```python
from build123d import *

# Parameters (mm, degrees)
F1_DEPTH  = 25.4
F2_R      = 6.2243902107
F2_R_2    = 6.3495156859
F3_DEPTH  = 12.701
F6_DEPTH  = 12.701
F8_DEPTH  = 12.701
F10_DEPTH = 12.701
F11_DEPTH = 12.701
F12_DEPTH = 12.701


# Not quite as in the source:
# - a feature names something its author has since deleted; it is built from what else it names


with BuildPart() as f1:
    # F0 (on Front) → F1 (new body)
    with BuildSketch(Plane.XZ):
        Polygon((-18.3063060958, 44.45), (-31.0063060958, 44.45), (-31.0063060958, 0), (26.1436939042, 0), (26.1436939042, 12.7), (-18.3063060958, 12.7), align=None)
    extrude(amount=F1_DEPTH)

    # F2 (on face) → F3 (cut, through all)
    with BuildSketch(Plane.XY.offset(12.7)):
        with Locations((-5.6063060958, -12.7)):
            Circle(F2_R)
        with Locations((13.4436939042, -12.7)):
            Circle(F2_R_2)
    extrude(amount=-F3_DEPTH, mode=Mode.SUBTRACT)

    # F4 (on face) → F6 (cut, through all)
    with BuildSketch(Plane.XY.offset(12.7)):
        with BuildLine():
            ThreePointArc((13.4436939042, 0), (22.4239500253, -3.7197438789), (26.1436939042, -12.7))
            Line((26.1436939042, -12.7), (26.1436939042, 0))
            Line((26.1436939042, 0), (13.4436939042, 0))
        make_face()
        with BuildLine():
            ThreePointArc((26.1436939042, -12.7), (22.4239500253, -21.6802561211), (13.4436939042, -25.4))
            Line((13.4436939042, -25.4), (26.1436939042, -25.4))
            Line((26.1436939042, -25.4), (26.1436939042, -12.7))
        make_face()
    extrude(amount=-F6_DEPTH, mode=Mode.SUBTRACT)

    # F7 (on face) → F8 (cut, through all)
    with BuildSketch(Plane.YZ.offset(-18.3063060958)):
        with BuildLine():
            ThreePointArc((-12.7, 44.45), (-3.7197438789, 40.7302561211), (0, 31.75))
            Line((0, 31.75), (0, 44.45))
            Line((0, 44.45), (-12.7, 44.45))
        make_face()
        with BuildLine():
            ThreePointArc((-25.4, 31.75), (-21.6802561211, 40.7302561211), (-12.7, 44.45))
            Line((-12.7, 44.45), (-25.4, 44.45))
            Line((-25.4, 44.45), (-25.4, 31.75))
        make_face()
    extrude(amount=-F8_DEPTH, mode=Mode.SUBTRACT)

    # F9 (on face) → F10 (cut, through all)
    with BuildSketch(Plane.YZ.offset(-18.3063060958)):
        with BuildLine():
            ThreePointArc((-12.7, 44.45), (-15.9870018728, 44.0172579939), (-19.05, 42.7485226281))
            Line((-19.05, 42.7485226281), (-19.05, 30.0485226281))
            ThreePointArc((-19.05, 30.0485226281), (-12.7, 23.6985226281), (-6.35, 30.0485226281))
            Line((-6.35, 30.0485226281), (-6.35, 42.7485226281))
            ThreePointArc((-6.35, 42.7485226281), (-9.4129981272, 44.0172579939), (-12.7, 44.45))
        make_face()
    extrude(amount=-F10_DEPTH, mode=Mode.SUBTRACT)

    # F7 (on face) → F11 (cut, through all)
    with BuildSketch(Plane.YZ.offset(-18.3063060958)):
        with BuildLine():
            ThreePointArc((-12.7, 44.45), (-3.7197438789, 40.7302561211), (0, 31.75))
            Line((0, 31.75), (0, 44.45))
            Line((0, 44.45), (-12.7, 44.45))
        make_face()
    extrude(amount=-F11_DEPTH, mode=Mode.SUBTRACT)

    # F7 (on face) → F12 (cut, through all)
    with BuildSketch(Plane.YZ.offset(-18.3063060958)):
        with BuildLine():
            ThreePointArc((-25.4, 31.75), (-21.6802561211, 40.7302561211), (-12.7, 44.45))
            Line((-12.7, 44.45), (-25.4, 44.45))
            Line((-25.4, 44.45), (-25.4, 31.75))
        make_face()
        with BuildLine():
            ThreePointArc((-12.7, 44.45), (-3.7197438789, 40.7302561211), (0, 31.75))
            Line((0, 31.75), (0, 44.45))
            Line((0, 44.45), (-12.7, 44.45))
        make_face()
    extrude(amount=-F12_DEPTH, mode=Mode.SUBTRACT)


solid = f1.part
```
Design review of the part built by this model. Coordinates are the model's own, in mm. A direction names the side the tool comes from. Give positions to 0.01 mm unless a question says otherwise; leave off trailing zeros. Loops run counter-clockwise (first coordinate to the right, second up) from the corner with the lowest first, then second, coordinate; pieces in that order, holes last. Notation, with made-up numbers: M 5,81.25 L 20,81.25 A25 ccw 20,115.25 Z; hole C 43.5,85 d9. An arc over 180 degrees is marked long. Return JSON: item names as keys, results as strings. Group by question number.
Item 1: We need section C-C (x = -9.5). Give the boundary of the cut face in (y, z).
Item 2: We need section B-B (z = 7). Give the boundary of the cut face in (x, y).
Item 3: Tool access review of faces 5 (the flat face through (4, -13, 12.7)), 6 (the cylindrical face through (16.86, -7.35, 6.44)), 7 (the flat face through (-25, -6.35, 36)): name each direction out of +Z, -Z, +X, -X, +Y, -Y from which nothing blocks a thin tool from reaching the whole face with its end or side.
Item 4: Insertion check: pin 1 Ø8 at (x, y) = (-24, -21.5) entering from -Z; pin 2 Ø7.5 at (x, y) = (0, -14) entering from +Z; pin 3 Ø10 at (y, z) = (-3.5, 38.5) entering from +X; pin 4 Ø5 at (x, y) = (-9, -11.5) entering from +Z. Each pin has a flat end and moves straight along its axis. Give the tip position at first contact, or say it passes through.
Item 5: We need section D-D (x = -20.5). Give the boundary of the cut face in (y, z), and give its area (3 significant figures).
Item 6: Mouldability with a two-part tool opening along X and no side actions: class faces 1 (the flat face through (-14, -25.4, 9)), 2 (the flat face through (-31.006, -13, 17)), 3 (the cylindrical face through (-10.2, -8.5, 6.4)), 4 (the flat face through (-18.306, -13, 21)) as released by +X, released by -X, zero draft, split by the parting line, or undercut.
Item 7: We need section A-A (y = -9.5). Give the boundary of the cut face in (x, z), and give its area (3 significant figures).
Item 8: For probe 1 along X at (y, z) = (-14, 7.5); probe 2 along Y at (x, z) = (-24, 30.5); probe 3 along X at (y, z) = (-1, 27), list the stretches that pass through material, from the lowest coordinate up.
Output:
{
 "1": {"outline": "M -25.4,0 L -17.56,0 L -17.56,12.7 L -25.4,12.7 Z; M -7.84,0 L 0,0 L 0,12.7 L -7.84,12.7 Z"},
 "2": {"outline": "M -31.01,-25.4 L 13.44,-25.4 A12.7 ccw 13.44,0 L -31.01,0 Z; hole C -5.61,-12.7 d12.45; hole C 13.44,-12.7 d12.7"},
 "3": {"face 5": "+Z, +X, +Y, -Y", "face 6": "+Z, -Z", "face 7": "+Z, +X, -X"},
 "4": {"pin 1": "stops at z = 0", "pin 2": "stops at z = 12.7", "pin 3": "stops at x = -18.31", "pin 4": "passes through"},
 "5": {"outline": "M -25.4,0 L 0,0 L 0,31.75 A12.7 ccw -6.35,42.75 L -6.35,30.05 A6.35 cw -19.05,30.05 L -19.05,42.75 A12.7 ccw -25.4,31.75 Z", "area": "821 mm^2"},
 "6": {"face 1": "zero draft", "face 2": "released by -X", "face 3": "undercut", "face 4": "released by +X"},
 "7": {"outline": "M -31.01,0 L -10.95,0 L -10.95,12.7 L -18.31,12.7 L -18.31,24.56 L -31.01,24.56 Z; M -0.27,0 L 7.96,0 L 7.96,12.7 L -0.27,12.7 Z; M 18.93,0 L 25.73,0 L 25.73,12.7 L 18.93,12.7 Z", "area": "596 mm^2"},
 "8": {"probe 1": "x = -31.01 to -11.69, 0.48 to 7.23, 19.66 to 26.08", "probe 2": "y = -25.4 to -19.05, -6.35 to 0", "probe 3": "x = -31.01 to -18.31"}
}
